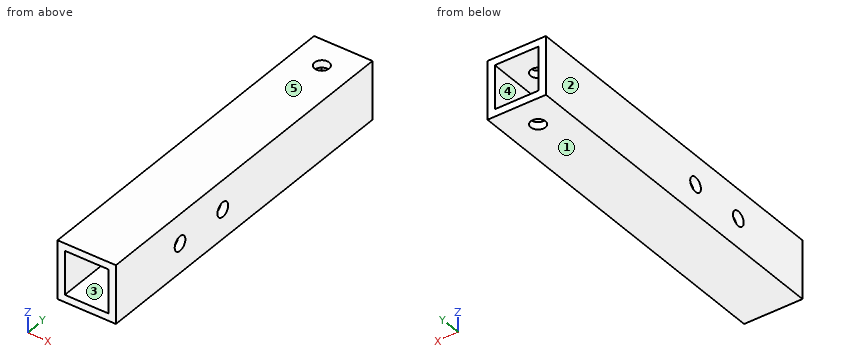
Autodesk Inventor part; units mm, degrees
ref_plane "YZ Plane" through (0, 0, 0) normal (1, 0, 0) x (0, 1, 0)
ref_plane "XZ Plane" through (0, 0, 0) normal (0, 1, 0) x (-1, 0, 0)
ref_plane "XY Plane" through (0, 0, 0) normal (0, 0, 1) x (1, 0, 0)
sketch "Sketch1" plane through (0, 0, 0) normal (0, 1, 0) x (-1, 0, 0)
  line L0 (0, 0) -> (25.4, 0)
  line L1 (25.4, 0) -> (25.4, 25.4)
  line L2 (25.4, 25.4) -> (0, 25.4)
  line L3 (0, 25.4) -> (0, 0)
  line L4 (22.225, 22.225) -> (3.175, 22.225)
  line L5 (3.175, 22.225) -> (3.175, 3.175)
  line L6 (3.175, 3.175) -> (22.225, 3.175)
  line L7 (22.225, 3.175) -> (22.225, 22.225)
  dimension "d0" = 25.4
  dimension "d1" = 25.4
  dimension "d4" = 3.175
  dimension "d5" = 3.175
  dimension "d7" = 3.175
  dimension "d8" = 3.175
extrude "Extrusion1" add sketch "Sketch1" along normal blind 152.4
sketch "Sketch2" plane through (-25.4, 0, 25.4) normal (0, 0, 1) x (1, 0, 0)
  circle A0 centre (12.7, 139.7) radius 3.175
  line L0 (0, 152.4) -> (25.4, 152.4)
  line L1 (0, 0) -> (0, 152.4)
  point P0 (25.4, 0)
  dimension "d11" = 6.35
  dimension "d12" = 12.7
  dimension "d13" = 12.7
extrude "Extrusion2" cut sketch "Sketch2" against normal through all
sketch "Sketch5" plane through (-25.4, 0, 0) normal (-1, 0, 0) x (0, 0, 1)
  circle A0 centre (12.7, 38.1) radius 3.175
  circle A1 centre (12.7, 63.5) radius 3.175
  line L0 (0, 0) -> (25.4, 0)
  line L1 (0, 0) -> (0, 152.4)
  dimension "d32" = 38.1
  dimension "d33" = 25.4
  dimension "d34" = 12.7
  dimension "d35" = 12.7
  dimension "d36" = 6.35
  dimension "d37" = 6.35
extrude "Extrusion5" cut sketch "Sketch5" against normal blind 25.4
properties part number "15102898-16-P-0505" material "Aluminum 6061"
Design review of the part built by this model. Coordinates are the model's own, in mm. Face numbers are marked on the shaded views. A direction names the side the tool comes from. Round coordinates to 2 decimals unless told otherwise and drop trailing zeros. Loops run counter-clockwise (first coordinate to the right, second up) from the corner with the lowest first, then second, coordinate; pieces in that order, holes last. Notation, with made-up numbers: M 71,31 L 105,31 A6 ccw 105,42 Z; hole C 22.5,63.25 d9. An arc over 180 degrees is marked long. Answer as a JSON object with one key per item and string values.
Item 1: The part is to be moulded in two halves that separate along Z. For the marked faces 1, 2 and 3, say which applies: pulls with the +Z half, pulls with the -Z half, needs draft (parallel to the pull), parting line crosses it, or undercut.
Answer sheet:
{"face 1": "pulls with the -Z half", "face 2": "needs draft", "face 3": "undercut"}
Item 2: We need section A-A on x = -12.7. Give the boundary of the cut face in (y, z) (3 decimals).
Answer sheet:
{"outline": "M 0,0 L 136.525,0 L 136.525,3.175 L 0,3.175 Z; M 0,22.225 L 136.525,22.225 L 136.525,25.4 L 0,25.4 Z; M 142.875,0 L 152.4,0 L 152.4,3.175 L 142.875,3.175 Z; M 142.875,22.225 L 152.4,22.225 L 152.4,25.4 L 142.875,25.4 Z"}
Item 3: We need section B-B on y = 38.1. Give the boundary of the cut face in (x, z) (3 decimals).
Answer sheet:
{"outline": "M -25.4,0 L 0,0 L 0,9.525 L -3.175,9.525 L -3.175,3.175 L -22.225,3.175 L -22.225,9.525 L -25.4,9.525 Z; M -25.4,15.875 L -22.225,15.875 L -22.225,22.225 L -3.175,22.225 L -3.175,15.875 L 0,15.875 L 0,25.4 L -25.4,25.4 Z"}
Item 4: Machinability: for the marked faces 4 and 5, which of the approach directions +Z, -Z, +X, -X, +Y, -Y give a long, thin tool a straight path to every point of the face, cutting with its end or side? Answer none if there is none.
Answer sheet:
{"face 4": "+Y, -Y", "face 5": "+Z, +X, -X, +Y, -Y"}
Item 5: We need section D-D on z = 12.7. Give the boundary of the cut face in (x, y) (3 decimals), and give its area (3 significant figures).
Answer sheet:
{"outline": "M -25.4,0 L -22.225,0 L -22.225,34.925 L -25.4,34.925 Z; M -25.4,41.275 L -22.225,41.275 L -22.225,60.325 L -25.4,60.325 Z; M -25.4,66.675 L -22.225,66.675 L -22.225,152.4 L -25.4,152.4 Z; M -3.175,0 L 0,0 L 0,34.925 L -3.175,34.925 Z; M -3.175,41.275 L 0,41.275 L 0,60.325 L -3.175,60.325 Z; M -3.175,66.675 L 0,66.675 L 0,152.4 L -3.175,152.4 Z", "area": "887 mm^2"}
Item 6: We need section C-C on x = -19.25. Give the boundary of the cut face in (y, z) (3 decimals).
Answer sheet:
{"outline": "M 0,0 L 152.4,0 L 152.4,3.175 L 0,3.175 Z; M 0,22.225 L 152.4,22.225 L 152.4,25.4 L 0,25.4 Z"}
Item 7: Wall thickness on L1, parallel to Y at x = -24.55, z = 12.7 (3 decimals); L2, parallel to X at y = 139.7, z = 1.85 (3 decimals); L3, parallel to Z at x = -14, y = 124.5 (3 decimals): over which ranges is each line inside the solid? List them lowest first. Write a range as from..to.
Answer sheet:
{"L1": "y = 0..34.925, 41.275..60.325, 66.675..152.4", "L2": "x = -25.4..-15.875, -9.525..0", "L3": "z = 0..3.175, 22.225..25.4"}
Item 8: Clearance check with flat-ended pins moving along their axes: P1, Ø6, axis at x = -20, z = 3.5, coming from the +Y side; P2, Ø5, axis at x = -12.7, y = 139.7, coming from the -Z side. State where each tip first meets the part, or that it passes through.
Answer sheet:
{"P1": "stops at y = 152.4", "P2": "passes through"}
